Build history of the part. All positions in model axes, mm. Give positions to 0.01 mm unless a question says otherwise; leave off trailing zeros. Order: outer loops, then holes, each group sorted by start corner. A loop starts at its lowest first (then second) coordinate and runs counter-clockwise, first axis right, second up. Notation, with made-up numbers: (86.5, 31.25) - (98.5, 31.25) arc R24 cw to (98.5, 58.25) - close; hole circle Ø2 at (-23, -13). An arc over 180 degrees is marked (long way). Use a Markdown table: item, result.
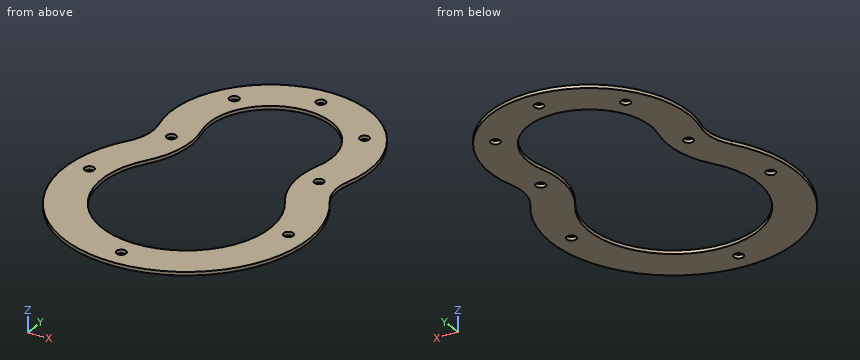
from build123d import *

# Parameters (mm, degrees)
BOSS_EXTRUDE1_DEPTH = 0.9
M3_TAPPED_HOLE1_D   = 2.5


with BuildPart() as part:
    # Sketch1 → Boss-Extrude1 (new body)
    with BuildSketch(Plane.XY):
        with BuildLine():
            ThreePointArc((-24.993351584, 27.835338346), (-24.67461016, 22.663230671), (-26.566359725, 17.838961039))
            ThreePointArc((-26.566359725, 17.838961039), (0, -32), (26.566359725, 17.838961039))
            ThreePointArc((26.566359725, 17.838961039), (24.67461016, 22.663230671), (24.993351584, 27.835338346))
            ThreePointArc((24.993351584, 27.835338346), (0, 61), (-24.993351584, 27.835338346))
        make_face()
        with BuildLine():
            ThreePointArc((-15.380524051, 30.590977444), (0, 51), (15.380524051, 30.590977444))
            ThreePointArc((15.380524051, 30.590977444), (14.796164774, 21.108780039), (18.264372311, 12.264285714))
            ThreePointArc((18.264372311, 12.264285714), (0, -22), (-18.264372311, 12.264285714))
            ThreePointArc((-18.264372311, 12.264285714), (-14.796164774, 21.108780039), (-15.380524051, 30.590977444))
        make_face(mode=Mode.SUBTRACT)
    extrude(amount=BOSS_EXTRUDE1_DEPTH)

    # M3 Tapped Hole1 (through all)
    with Locations(Plane.XY.offset(0.9)):
        with Locations((27, 0), (19.528744622, 24.528571429), (-19.528744622, 24.528571429), (-26.92368656, 2.028571429), (0, 56), (17.213758142, 47.028571429), (-17.213758142, 47.028571429), (0, -27)):
            Hole(M3_TAPPED_HOLE1_D / 2)


solid = part.part
1) Slice it at B-B (y = -27). Write the cut outline in (x, z), and give its area (3 significant figures).
Computed:
| item | result |
|---|---|
| outline | (-17.18, 0) - (-1.25, 0) - (-1.25, 0.9) - (-17.18, 0.9) - close; (1.25, 0) - (17.18, 0) - (17.18, 0.9) - (1.25, 0.9) - close |
| area | 28.7 mm² |
2) Slice it at C-C (z = 0.65). State how many separate pieces and enclosed holes the cut face has, and give its area (3 significant figures).
Computed:
| item | result |
|---|---|
| separate pieces | 1 |
| enclosed holes | 9 |
| area | 2,200 mm² |
3) Slice it at D-D (x = -19.5). Write the cut outline in (y, z), and give its area (3 significant figures).
Computed:
| item | result |
|---|---|
| outline | (-25.37, 0) - (-10.19, 0) - (-10.19, 0.9) - (-25.37, 0.9) - close; (10.19, 0) - (23.28, 0) - (23.28, 0.9) - (10.19, 0.9) - close; (25.78, 0) - (52.2, 0) - (52.2, 0.9) - (25.78, 0.9) - close |
| area | 49.2 mm² |
4) Wall check: line 1 (X direction, y = 24.5, z = 0.8); line 2 (Y direction, x = -1, z = 0.65); line 3 (X direction, y = 35, z = 0.7). Give the ranges that are in metal, low to high. Write a range as from..to.
Computed:
| item | result |
|---|---|
| line 1 | x = -24.53..-20.78, -18.28..-14.53, 14.53..18.28, 20.78..24.53 |
| line 2 | y = -31.98..-27.75, -26.25..-21.98, 50.97..55.25, 56.75..60.98 |
| line 3 | x = -26..-16, 16..26 |
5) Slice it at A-A (x = 0). Write the cut outline in (y, z).
Computed:
| item | result |
|---|---|
| outline | (-32, 0) - (-28.25, 0) - (-28.25, 0.9) - (-32, 0.9) - close; (-25.75, 0) - (-22, 0) - (-22, 0.9) - (-25.75, 0.9) - close; (51, 0) - (54.75, 0) - (54.75, 0.9) - (51, 0.9) - close; (57.25, 0) - (61, 0) - (61, 0.9) - (57.25, 0.9) - close |
6) Pin check, flat tip, straight feed: P1, Ø3, axis at x = 0, y = 56, coming from the +Z side. Stop position of the tip, or through.
Computed:
| item | result |
|---|---|
| P1 | stops at z = 0.9 |
